Check sheet for the modelled part. Datum: model origin and axes. Units: mm. Face numbers are marked on the shaded views. A direction names the side the tool comes from. Coordinates: 2 decimals unless noted, no trailing zeros. Loops run counter-clockwise (first coordinate to the right, second up) from the corner with the lowest first, then second, coordinate; pieces in that order, holes last. Notation, with made-up numbers: M 20,5 L 75,5 A23 cw 75,22 Z; hole C 30,72 d3. An arc over 180 degrees is marked long. Write each question's results on one line, items separated by ' | '. Start each with the question number.
from build123d import *

# Parameters (mm, degrees)
SKETCH_1_W          = 20
SKETCH_1_H          = 10
EXTRUDE_1_DEPTH     = 4.5
CUT_EXTRUDE_1_DEPTH = 4.5
EXTRUDE_2_DEPTH     = 4.5
SKETCH_5_W          = 3
SKETCH_5_H          = 3
CUT_EXTRUDE_2_DEPTH = 4.5
SKETCH_6_W          = 3
SKETCH_6_H          = 4.5
EXTRUDE_3_DEPTH     = 11


with BuildPart() as part:
    # 草图1 → 凸台-拉伸1 (new body)
    with BuildSketch(Plane(origin=(0, 0, 0), x_dir=(1, 0, 0), z_dir=(0, 1, 0))):
        Rectangle(SKETCH_1_W, SKETCH_1_H)
    extrude(amount=EXTRUDE_1_DEPTH)

    # 草图2 → 切除-拉伸1 (cut)
    with BuildSketch(Plane(origin=(0, 4.5, 0), x_dir=(1, 0, 0), z_dir=(0, 1, 0))):
        with BuildLine():
            Line((-2.814231537, 3.495066534), (6.5, 3))
            Line((6.5, 3), (6.5, -3))
            Line((6.5, -3), (-2.814231537, -3.495066534))
            ThreePointArc((-2.814231537, -3.495066534), (-6.5, 0), (-2.814231537, 3.495066534))
        make_face()
    extrude(amount=-CUT_EXTRUDE_1_DEPTH, mode=Mode.SUBTRACT)

    # 草图3 → 凸台-拉伸2 (add)
    with BuildSketch(Plane(origin=(0, 4.5, 0), x_dir=(1, 0, 0), z_dir=(0, 1, 0))):
        with BuildLine():
            ThreePointArc((10, 5), (0, 11.180339887), (-10, 5))
            Line((-10, 5), (10, 5))
        make_face()
        with BuildLine():
            Line((-10, -5), (-10, 5))
            ThreePointArc((-10, 5), (-11.180339887, 0), (-10, -5))
        make_face()
        with BuildLine():
            Line((10, -5), (-10, -5))
            ThreePointArc((-10, -5), (0, -11.180339887), (10, -5))
        make_face()
        with BuildLine():
            ThreePointArc((11.180339887, 0), (10.881254497, 2.568715742), (10, 5))
            Line((10, 5), (10, -5))
            ThreePointArc((10, -5), (10.881254497, -2.568715742), (11.180339887, 0))
        make_face()
    extrude(amount=-EXTRUDE_2_DEPTH)

    # 草图5 → 切除-拉伸2 (cut)
    with BuildSketch(Plane(origin=(0, 4.5, 0), x_dir=(1, 0, 0), z_dir=(0, 1, 0))):
        with Locations((0, -9.680339887)):
            Rectangle(SKETCH_5_W, SKETCH_5_H)
    extrude(amount=-CUT_EXTRUDE_2_DEPTH, mode=Mode.SUBTRACT)

    # 草图6 → 凸台-拉伸3 (add)
    with BuildSketch(Plane.XY.offset(8.180339887)):
        with Locations((0, 2.25)):
            Rectangle(SKETCH_6_W, SKETCH_6_H)
    extrude(amount=EXTRUDE_3_DEPTH)


solid = part.part
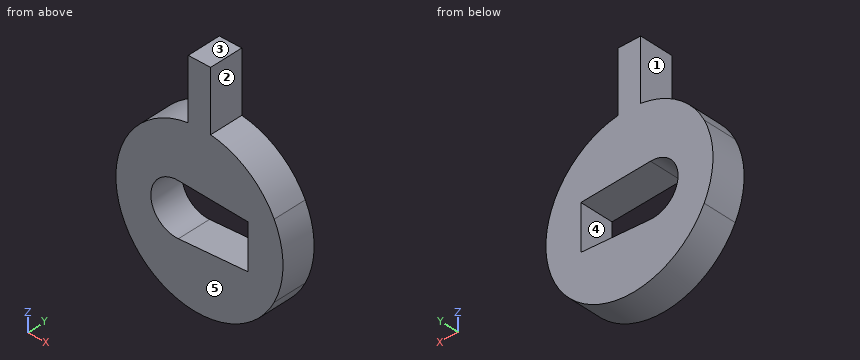
1) Section check B-B (y = 1.2). Enter the section's corners in (x, z).
2) Section check D-D (z = 12). Enter the section's corners in (x, y).
3) Section check C-C (x = 2.5). Enter the section's corners in (y, z), then the cut area to 3 significant figures.
4) Thickness scan on probe 1 along Z at (x, y) = (-3.25, 3.25); probe 2 along Z at (x, y) = (5.5, 1.2); probe 3 along X at (y, z) = (1.3, 16). Record the ranges inside material, lowest first.
5) Gauge pin test, flat ends, axial feed: P1, Ø1, axis at x = -0.5, z = -5.5, coming from the -Y side; P2, Ø1.3, axis at y = 1.5, z = 15.5, coming from the -X side; P3, Ø1.3, axis at y = 3, z = 1, coming from the -X side. Record the tip position at first contact, or that the pin passes through.
6) Set-up check for the marked faces 1, 2, 3, 4 and 5: record each of +Z, -Z, +X, -X, +Y, -Y from which the full face is reachable in a straight line by a thin tool's end or side.
7) Section check A-A (z = 0). Enter the section's corners in (x, y), then the cut area to 3 significant figures.
Return value:
1) outline: M -1.5,11.08 A11.18 ccw long 1.5,11.08 L 1.5,19.18 L -1.5,19.18 Z; hole M -2.81,-3.5 L 6.5,-3 L 6.5,3 L -2.81,3.5 A3.5 ccw long Z
2) outline: M -1.5,0 L 1.5,0 L 1.5,4.5 L -1.5,4.5 Z
3) outline: M 0,-10.9 L 4.5,-10.9 L 4.5,-3.21 L 0,-3.21 Z; M 0,3.21 L 4.5,3.21 L 4.5,10.9 L 0,10.9 Z | area: 69.2 mm2
4) probe 1: z = -10.7 to -3.49, 3.49 to 10.7 | probe 2: z = -9.73 to -3.05, 3.05 to 9.73 | probe 3: x = -1.5 to 1.5
5) P1: stops at y = 0 | P2: stops at x = -1.5 | P3: stops at x = -11.17
6) face 1: +Z, -X, +Y, -Y | face 2: +Z, +X, +Y, -Y | face 3: +Z, +X, -X, +Y, -Y | face 4: +Y, -Y | face 5: +Z, -Z, +X, -X, -Y
7) outline: M -11.18,0 L -6.5,0 L -6.5,4.5 L -11.18,4.5 Z; M 6.5,0 L 11.18,0 L 11.18,4.5 L 6.5,4.5 Z | area: 42.1 mm2
